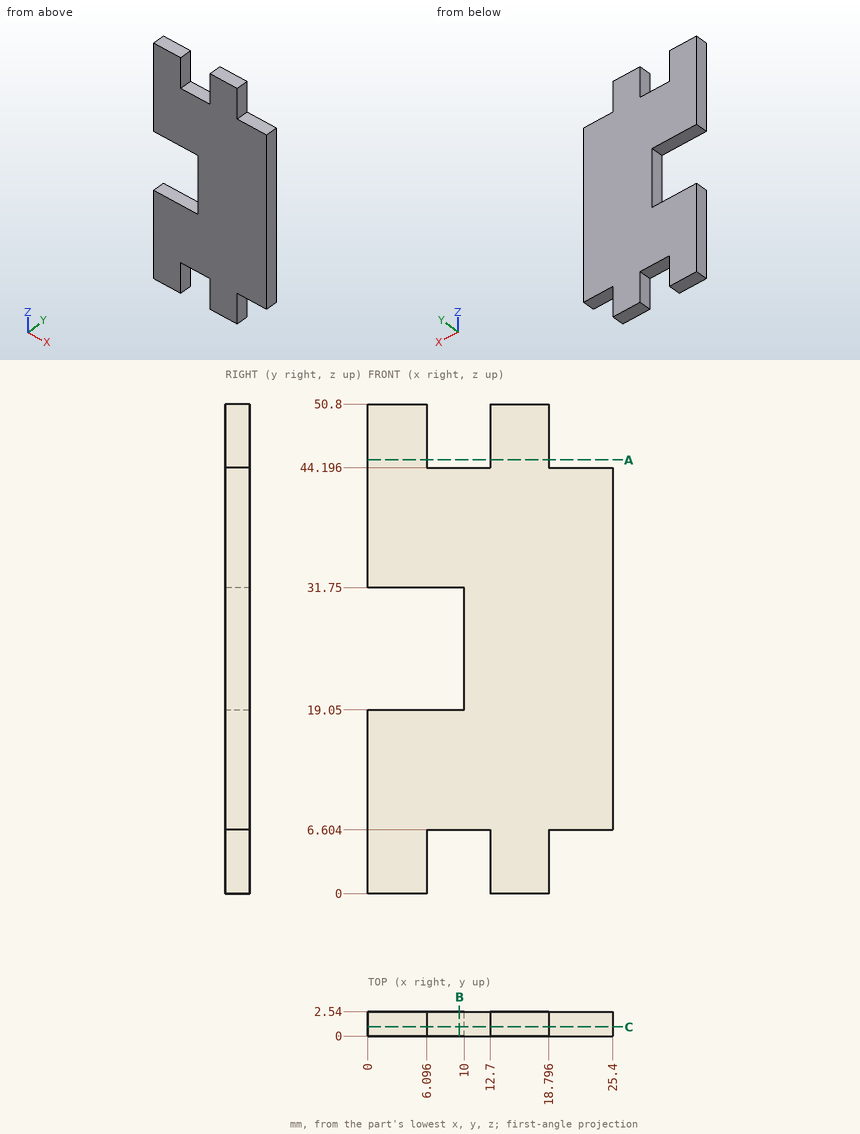
Verification items for this drawing (mm, ordinates from the low corner). Coordinates: 2 decimals unless noted, no trailing zeros. Write each loop counter-clockwise with the first axis right and the second up, starting at its lowest first coordinate (ties: lowest second). Pieces come first, ordered by that corner, then holes. Notation, with made-up numbers: M 4,14.5 L 26,14.5 A23 cw 26,45.5 Z; hole C -19.5,-10.5 d8. An arc over 180 degrees is marked long. One line per item, written item: value. Start each with the question number.
(1) Sectioned sample at C-C, the plane y = 0.95. Enter the section's corners in (x, z), and give its area (3 significant figures).
(2) Sectioned sample at A-A, the plane z = 45. Enter the section's corners in (x, y), and give its area (3 significant figures).
(3) Scan lines: line 1 along Z through (x, y) = (6.25, 1.45); line 2 along X through (y, z) = (0.3, 45.5); line 3 along Z through (x, y) = (5.25, 0.85). Record each from-to range of solid material in increasing order. Write a range as [from, to].
(4) Sectioned sample at B-B, the plane x = 9.5. Enter the section's corners in (y, z).
(5) Depth check by flat-ended pin: pin 1 (1.3 mm diameter, centred on y = 1, z = 3.5, fed in from +X); pin 2 (0.8 mm diameter, centred on y = 1, z = 26, fed in from -X); pin 3 (0.8 mm diameter, centred on x = 9, y = 1, fed in from -Z). Enter the tip coordinate at first touch or a pass-through.
Filled sheet:
1. outline: M 0,0 L 6.1,0 L 6.1,6.6 L 12.7,6.6 L 12.7,0 L 18.8,0 L 18.8,6.6 L 25.4,6.6 L 25.4,44.2 L 18.8,44.2 L 18.8,50.8 L 12.7,50.8 L 12.7,44.2 L 6.1,44.2 L 6.1,50.8 L 0,50.8 L 0,31.75 L 10,31.75 L 10,19.05 L 0,19.05 Z
1. area: 989 mm²
2. outline: M 0,0 L 6.1,0 L 6.1,2.54 L 0,2.54 Z; M 12.7,0 L 18.8,0 L 18.8,2.54 L 12.7,2.54 Z
2. area: 31.0 mm²
3. line 1: [6.6, 19.05], [31.75, 44.2]
3. line 2: [0, 6.1], [12.7, 18.8]
3. line 3: [0, 19.05], [31.75, 50.8]
4. outline: M 0,6.6 L 2.54,6.6 L 2.54,19.05 L 0,19.05 Z; M 0,31.75 L 2.54,31.75 L 2.54,44.2 L 0,44.2 Z
5. pin 1: x = 18.8
5. pin 2: x = 10
5. pin 3: z = 6.6
